from build123d import *

# Parameters (mm, degrees)
SKETCH1_R           = 70.75
SKETCH1_W           = 121.5
SKETCH1_H           = 44.787071271
BOSS_EXTRUDE1_DEPTH = 50
SKETCH2_R           = 1.5
SKETCH2_R_2         = 2.55
CUT_EXTRUDE1_DEPTH  = 5
CIRPATTERN1_COUNT   = 3


with BuildPart() as part:
    # Sketch1 → Boss-Extrude1 (new body)
    with BuildSketch(Plane(origin=(0, 0, 0), x_dir=(1, 0, 0), z_dir=(0, 1, 0))):
        Circle(SKETCH1_R)
        with Locations((0, -58.656464365)):
            Rectangle(SKETCH1_W, SKETCH1_H)
    extrude(amount=BOSS_EXTRUDE1_DEPTH)

    # Sketch2 → Cut-Extrude1 (cut)
    with BuildSketch(Plane(origin=(0, 0, 0), x_dir=(-1, 0, 0), z_dir=(0, -1, 0))):
        with Locations(Location((0, 50, 0), (0, 0, 90))):
            Circle(SKETCH2_R)
        with Locations(Location((0, 0, 0), (0, 0, 90))):
            Circle(SKETCH2_R_2)
    cut_extrude1 = extrude(amount=-CUT_EXTRUDE1_DEPTH, mode=Mode.SUBTRACT)

    # CirPattern1: Cut-Extrude1 ×3 about axis
    cirpattern1_axis = Axis((0, 0, 0), (0, 1, 0))
    for i in range(1, CIRPATTERN1_COUNT):
        add(cut_extrude1.rotate(cirpattern1_axis, i * 360 / CIRPATTERN1_COUNT), mode=Mode.SUBTRACT)


solid = part.part
The listing builds one solid part. Answer for the finished solid, in the listing's coordinates (mm). A direction names the side the tool comes from. Round coordinates to 2 decimals unless told otherwise and drop trailing zeros. Write each loop counter-clockwise with the first axis right and the second up, starting at its lowest first coordinate (ties: lowest second). Pieces come first, ordered by that corner, then holes. Notation, with made-up numbers: (60, 42.5) - (92, 42.5) arc R7 ccw to (92, 49.5) - close; hole circle Ø11 at (2, -24.75). An arc over 180 degrees is marked (long way). Use a Markdown table: item, result. Add a question column.
1. Flat-ended cylindrical pins translate along their axes: P1, Ø1.5, axis at x = -0.5, z = -0.5, coming from the -Y side; P2, Ø2.5, axis at x = -43, z = 25.5, coming from the -Y side; P3, Ø22.5, axis at y = 13, z = 48, coming from the -X side; P4, Ø5, axis at y = 22.5, z = -20.5, coming from the +X side. Find the tip coordinate at first contact, or state that the pin passes through.
2. Consider line 1 (X direction, y = 2.4, z = 0); line 2 (X direction, y = 1, z = 25); line 3 (Z direction, x = -48.5, y = 19). Determine where each line is inside the solid, lowest interval first.
3. The part is cut by section A-A (y = 29). Write down the section's boundary in (x, z), and give its area (3 significant figures).
4. For a pull along Z with two mould halves and no side action, classify faces 1 (the face through (-1, 0, 4)), 2 (the face through (2.09, 24.65, -70.72)), 3 (the face through (0, 5, 0)) as +Z half, -Z half, draft (parallel to the pull), parting line (faces both ways), or undercut.
5. The part is cut by section B-B (z = 16). Write down the section's boundary in (x, y), and give its area (3 significant figures).
6. A tool of negligible diameter and unlimited length cuts with its end or side. For faces 4 (the face through (-1, 25, 81.05)), 5 (the face through (-60.75, 25, 59)), 6 (the face through (0.77, 2.46, -2.43)), 7 (the face through (-1, 50, 4)), 8 (the face through (60.75, 25, 59)), from which of +Z, -Z, +X, -X, +Y, -Y can it reach the whole face along a straight path? Write none if from no direction.
Reported:
| question | item | result |
|---|---|---|
| 1 | P1 | y = 5 |
| 1 | P2 | y = 0 |
| 1 | P3 | x = -60.75 |
| 1 | P4 | x = 68.42 |
| 2 | line 1 | -70.75 to -2.55, 2.55 to 70.75 |
| 2 | line 2 | -66.19 to -44.8, -41.8 to 41.8, 44.8 to 66.19 |
| 2 | line 3 | -51.51 to 81.05 |
| 3 | outline | (-60.75, 36.26) arc R70.75 ccw (long way) to (60.75, 36.26) - (60.75, 81.05) - (-60.75, 81.05) - close |
| 3 | area | 18,200 mm^2 |
| 4 | face 1 | draft |
| 4 | face 2 | parting line |
| 4 | face 3 | undercut |
| 5 | outline | (-68.92, 0) - (68.92, 0) - (68.92, 50) - (-68.92, 50) - close |
| 5 | area | 6,890 mm^2 |
| 6 | face 4 | +Z, +X, -X, +Y, -Y |
| 6 | face 5 | +Z, -X, +Y, -Y |
| 6 | face 6 | -Y |
| 6 | face 7 | +Z, -Z, +X, -X, +Y |
| 6 | face 8 | +Z, +X, +Y, -Y |
